Here's how the part is built. I have some questions about the finished solid (model axes, mm). Round coordinates to 2 decimals unless told otherwise and drop trailing zeros. Loops run counter-clockwise (first coordinate to the right, second up) from the corner with the lowest first, then second, coordinate; pieces in that order, holes last. Notation, with made-up numbers: M -25,21.5 L 4,21.5 A23 cw 4,54.5 Z; hole C -24,-4.75 d5. An arc over 180 degrees is marked long. Write each question's results on one line, items separated by ' | '. Start each with the question number.
```python
from build123d import *

# Parameters (mm, degrees)
SKETCH1_W           = 139.192
SKETCH1_H           = 101.092
BASE_EXTRUDE_DEPTH  = 38.1
BOSS_EXTRUDE1_DEPTH = 0.762


with BuildPart() as part:
    # Sketch1 → Base-Extrude (new body)
    with BuildSketch(Plane.XY):
        with Locations((-5.306370086, 124.85517785)):
            Rectangle(SKETCH1_W, SKETCH1_H)
    extrude(amount=BASE_EXTRUDE_DEPTH)

    # Sketch2 → Boss-Extrude1 (add)
    with BuildSketch(Plane.XY.offset(38.1)):
        with BuildLine():
            Line((-71.194022628, 171.043454179), (61.725007309, 171.043454179))
            ThreePointArc((61.725007309, 171.043454179), (61.904612432, 170.969059301), (61.979007309, 170.789454179))
            Line((61.979007309, 170.789454179), (61.979007309, 138.411180808))
            ThreePointArc((61.979007309, 138.411180808), (61.904612432, 138.231575686), (61.725007309, 138.157180808))
            Line((61.725007309, 138.157180808), (-71.194022628, 138.157180808))
            ThreePointArc((-71.194022628, 138.157180808), (-71.373627751, 138.231575686), (-71.448022628, 138.411180808))
            Line((-71.448022628, 138.411180808), (-71.448022628, 170.789454179))
            ThreePointArc((-71.448022628, 170.789454179), (-71.373627751, 170.969059301), (-71.194022628, 171.043454179))
        make_face()
        with BuildLine():
            Line((45.473947187, 135.025154773), (61.409083872, 135.025154773))
            ThreePointArc((61.409083872, 135.025154773), (61.588688995, 134.950759895), (61.663083872, 134.771154773))
            Line((61.663083872, 134.771154773), (61.663083872, 131.364122229))
            ThreePointArc((61.663083872, 131.364122229), (61.588688995, 131.184517106), (61.409083872, 131.110122229))
            Line((61.409083872, 131.110122229), (45.473947187, 131.110122229))
            ThreePointArc((45.473947187, 131.110122229), (45.294342065, 131.184517106), (45.219947187, 131.364122229))
            Line((45.219947187, 131.364122229), (45.219947187, 134.771154773))
            ThreePointArc((45.219947187, 134.771154773), (45.294342065, 134.950759895), (45.473947187, 135.025154773))
        make_face()
        with BuildLine():
            Line((22.766758431, 135.025154773), (25.665790975, 135.025154773))
            ThreePointArc((25.665790975, 135.025154773), (25.845396098, 134.950759895), (25.919790975, 134.771154773))
            Line((25.919790975, 134.771154773), (25.919790975, 131.872122229))
            ThreePointArc((25.919790975, 131.872122229), (25.845396098, 131.692517106), (25.665790975, 131.618122229))
            Line((25.665790975, 131.618122229), (22.766758431, 131.618122229))
            ThreePointArc((22.766758431, 131.618122229), (22.587153309, 131.692517106), (22.512758431, 131.872122229))
            Line((22.512758431, 131.872122229), (22.512758431, 134.771154773))
            ThreePointArc((22.512758431, 134.771154773), (22.587153309, 134.950759895), (22.766758431, 135.025154773))
        make_face()
        with BuildLine():
            Line((30.596823519, 135.025154773), (33.495856063, 135.025154773))
            ThreePointArc((33.495856063, 135.025154773), (33.675461186, 134.950759895), (33.749856063, 134.771154773))
            Line((33.749856063, 134.771154773), (33.749856063, 131.872122229))
            ThreePointArc((33.749856063, 131.872122229), (33.675461186, 131.692517106), (33.495856063, 131.618122229))
            Line((33.495856063, 131.618122229), (30.596823519, 131.618122229))
            ThreePointArc((30.596823519, 131.618122229), (30.417218397, 131.692517106), (30.342823519, 131.872122229))
            Line((30.342823519, 131.872122229), (30.342823519, 134.771154773))
            ThreePointArc((30.342823519, 134.771154773), (30.417218397, 134.950759895), (30.596823519, 135.025154773))
        make_face()
    extrude(amount=BOSS_EXTRUDE1_DEPTH)


solid = part.part
```
1. For pin 1 (8 mm diameter, centred on x = -41, y = 125, fed in from +Z); pin 2 (0.6 mm diameter, centred on x = 25, z = 38.5, fed in from +Y); pin 3 (0.6 mm diameter, centred on x = 8.5, z = 38.5, fed in from -Y), each with a flat end and sliding along its axis, tell me the tip position at first contact or that it passes through.
2. I need wall thicknesses on line 1 along Z through (x, y) = (-52.5, 93). Which ranges of the line are inside material? Lowest first, please.
3. I want a section at A-A on y = 90.5. List the corners of the cut face in (x, z) for me.
Outcome:
1) pin 1: z = 38.1 | pin 2: y = 171.04 | pin 3: y = 138.16
2) line 1: 0 to 38.1
3) outline: M -74.9,0 L 64.29,0 L 64.29,38.1 L -74.9,38.1 Z
